CAD build for the part. Positions are in the model's coordinates, mm. Face numbers are marked on the shaded views. A direction names the side the tool comes from. Coordinates: 2 decimals unless noted, no trailing zeros. Loops run counter-clockwise (first coordinate to the right, second up) from the corner with the lowest first, then second, coordinate; pieces in that order, holes last. Notation, with made-up numbers: (62, 62) -> (103, 62) arc R21 ccw to (103, 99) -> close; hole circle Ø1 at (-19, -3). An arc over 180 degrees is marked (long way). Write each question's results on one line, items separated by ' | '.
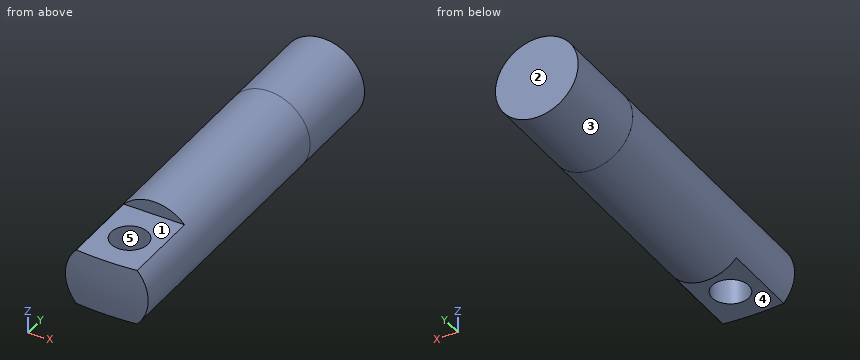
Solid Edge part; units mm, degrees
sketch "Sketch1" plane through (0, 0, 0) normal (0, -1, 0) x (1, 0, 0)
  circle A0 centre (0, 0) radius 4.5
extrude "Protrusion1" add sketch "Sketch1" along normal blind 30
sketch "Sketch2" plane through (0, 0, 3.05) normal (0, 0, 1) x (1, 0, 0)
  line L0 (-8.9921, -33.4091) -> (-8.9921, -21)
  line L1 (-8.9921, -21) -> (16.3275, -21)
  line L2 (16.3275, -21) -> (16.3275, -33.9732)
  line L3 (16.3275, -33.9732) -> (-8.9921, -33.4091)
extrude "Extrusionsausschnitt_1" cut sketch "Sketch2" along normal blind 50.5
mirror "Mirror1" about plane through (0, 0, 0) normal (0, 0, 1) of "Extrusionsausschnitt_1"
sketch "Sketch3" plane through (0, -25.5, 3.05) normal (0, 0, 1) x (0, 1, 0)
  circle A0 centre (0, 0) radius 2
extrude "Extrusionsausschnitt_2" cut sketch "Sketch3" against normal blind 11.5
sketch "Sketch4" plane through (0, 0, 0) normal (0, 0, 1) x (1, 0, 0)
  line L0 (4.661, -29.6509) -> (5.9893, -29.6509)
  arc A0 (0, -30) -> (4.661, -29.6509) centre (0, 1.2934) ccw
revolve "RevolvedCutout1" cut sketch "Sketch4" angle 360 about axis through (0, -30, 0) along (0, -1, 0) material side at (5.3252, -29.7009, 0)
sketch "Sketch5" plane through (0, 0, 0) normal (0, 1, 0) x (0, 0, -1)
  circle A0 centre (0, 0) radius 4.495
extrude "Protrusion2" add sketch "Sketch5" along normal blind 10
Q1. Pull direction X, two halves, no side cores. Call the marked faces 3, 4 and 5: +X half, -X half, draft (parallel to the pull), parting line (faces both ways), or undercut.
Results are:
face 3: parting line | face 4: draft | face 5: undercut
Q2. Cut at B-B on y = -25.5. Write the cut outline in (x, z), and give its area (3 significant figures).
Results are:
outline: (-3.31, -3.05) -> (-2, -3.05) -> (-2, 3.05) -> (-3.31, 3.05) arc R4.5 ccw to start; (2, -3.05) -> (3.31, -3.05) arc R4.5 ccw to (3.31, 3.05) -> (2, 3.05) -> close | area: 25.9 mm^2
Q3. Cut at A-A on x = 0. Write the cut outline in (y, z) (3 decimals), and give its area (3 significant figures).
Results are:
outline: (-29.851, -3.05) -> (-27.5, -3.05) -> (-27.5, 3.05) -> (-29.851, 3.05) arc R31.293 ccw to start; (-23.5, -3.05) -> (-21, -3.05) -> (-21, -4.5) -> (0, -4.5) -> (0, -4.495) -> (10, -4.495) -> (10, 4.495) -> (0, 4.495) -> (0, 4.5) -> (-21, 4.5) -> (-21, 3.05) -> (-23.5, 3.05) -> close | area: 309 mm^2
Q4. Which spindle directions (+Z, -Z, +X, -X, +Y, -Y) get a long thin tool onto all of the face, cutting with end or side? Do the marked faces 1 and 2. Say none if no direction does.
Results are:
face 1: +Z, +X, -X, -Y | face 2: +Z, -Z, +X, -X, +Y
Q5. Drop flat-ended pins along their axis: pin 1 (2 mm diameter, centred on y = 4.5, z = 2.5, fed in from +X); pin 2 (3 mm diameter, centred on x = -1, z = -2.5, fed in from -Y); pin 3 (1.6 mm diameter, centred on x = 1, z = 3.5, fed in from -Y). Give the stop position or say it passes through.
Results are:
pin 1: x = 4.24 | pin 2: y = -29.98 | pin 3: y = -29.87
Q6. Wall check: L1, parallel to Y at x = 0, z = 0.25; L2, parallel to Z at x = 0.25, y = 0.5; L3, parallel to Y at x = -1.75, z = 1 (3 decimals). Give the ranges that are in metal, low to high. Write a range as from..to.
Results are:
L1: -30..-27.5, -23.5..10 | L2: -4.49..4.49 | L3: -29.935..-26.468, -24.532..10
